Input: part model. Units: mm. Frame: model coordinates. A direction names the side the tool comes from. Coordinates: 2 decimals unless noted, no trailing zeros. Loops run counter-clockwise (first coordinate to the right, second up) from the corner with the lowest first, then second, coordinate; pieces in that order, holes last. Notation, with made-up numbers: M 9,87.25 L 49,87.25 A23 ccw 49,123.25 Z; hole C -13,85.25 d11. An arc over 180 degrees is marked long. Use a Markdown table: item, result. Add a question column.
1. Line query: L1, parallel to Y at x = 1.5, z = 17; L2, parallel to X at y = 0.75, z = 24. Output: solid intervals per line, ascending. Write a range as [from, to].
2. Section A-A on z = 29. Output: boundary loops of the cut face in (x, y).
3. Section B-B on x = 0. Output: boundary loops of the cut face in (y, z), then the cut area to 4 significant figures.
4. Pin query (flat end, axial travel): pin 1 (2 mm diameter, centred on x = -1, y = 1, fed in from -Z); pin 2 (5 mm diameter, centred on x = 2, z = 27.5, fed in from -Y); pin 3 (1 mm diameter, centred on y = -2, z = 19.5, fed in from +X); pin 4 (0.6 mm diameter, centred on x = 0, z = 23, fed in from +Y). Return the tip coordinate at first contact, or that it passes through.
5. Set-up query: faces 1 (the flat face through (1, 2, 23)), 2 (the flat face through (-2, 1, 23)), 3 (the flat face through (2, -1, 23)), 4 (the flat face through (-1, -2, 23)). Return all of +Z, -Z, +X, -X, +Y, -Y with unobstructed straight access to the full face (end or side cutting, diameter ignored); none if empty.
Autodesk Fusion 360 part; units mm, degrees
sketch "Sketch1" plane through (0, 0, 0) normal (0, 0, 1) x (1, 0, 0)
  circle A0 centre (0, 0) radius 3.75
  dimension "d1" = 7.5
extrude "Extrude1" add sketch "Sketch1" along normal blind 11
sketch "Sketch2" plane through (0, 0, 11) normal (0, 0, 1) x (-1, 0, 0)
  circle A0 centre (0, 0) radius 3.75
  circle A1 centre (0, 0) radius 4.5
  dimension "d4" = 9
extrude "Extrude2" add sketch "Sketch2" along normal blind 2 contours A0 | A1
sketch "Sketch3" plane through (0, 0, 13) normal (0, 0, 1) x (-1, 0, 0)
  circle A0 centre (0, 0) radius 4.5
  line L0 (-1, 3) -> (1, 3)
  line L1 (1, -3) -> (-1, -3)
  line L2 (-3, 1) -> (-3, -1)
  line L3 (3, -1) -> (3, 1)
  line L4 (3, 1) -> (1, 1)
  line L5 (-1, 1) -> (-3, 1)
  line L6 (-1, -3) -> (-1, -1)
  line L7 (-1, 1) -> (-1, 3)
  line L8 (1, 3) -> (1, 1)
  line L9 (1, -1) -> (1, -3)
  line L10 (-3, -1) -> (-1, -1)
  line L11 (1, -1) -> (3, -1)
  dimension "d7" = 6
  dimension "d8" = 6
  dimension "d9" = 2
extrude "Extrude3" add sketch "Sketch3" along normal blind 21 contours L0 L1 L2 L3 L4 L5 L6 L7 L8 L9 L10 L11
Answers below:
| question | item | result |
|---|---|---|
| 1 | L1 | y = [-1, 1] |
| 1 | L2 | x = [-3, 3] |
| 2 | outline | M -3,-1 L -1,-1 L -1,-3 L 1,-3 L 1,-1 L 3,-1 L 3,1 L 1,1 L 1,3 L -1,3 L -1,1 L -3,1 Z |
| 3 | outline | M -4.5,11 L -3.75,11 L -3.75,0 L 3.75,0 L 3.75,11 L 4.5,11 L 4.5,13 L 3,13 L 3,34 L -3,34 L -3,13 L -4.5,13 Z |
| 3 | area | 226.5 mm² |
| 4 | pin 1 | stops at z = 0 |
| 4 | pin 2 | stops at y = -3 |
| 4 | pin 3 | stops at x = 1 |
| 4 | pin 4 | stops at y = 3 |
| 5 | face 1 | +Z, +X, +Y |
| 5 | face 2 | +Z, -X, +Y |
| 5 | face 3 | +Z, +X, -Y |
| 5 | face 4 | +Z, -X, -Y |
